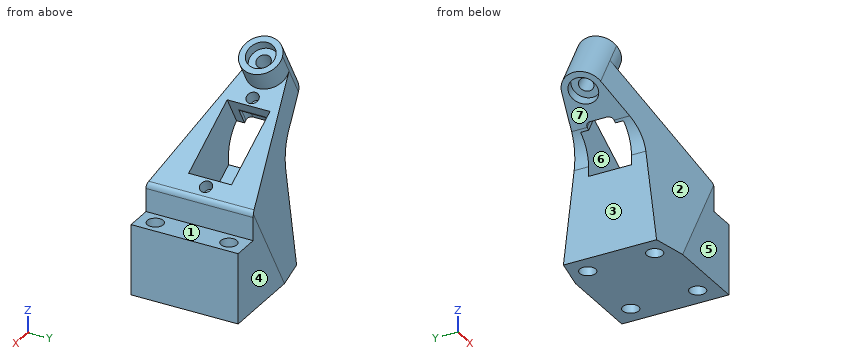
Autodesk Fusion 360 part; units mm, degrees
sketch "Main" plane through (0, 0, 0) normal (0, 1, 0) x (1, 0, 0)
  line L0 (0, 0) -> (35, 0)
  line L1 (35, 0) -> (35, -21)
  line L2 (-19.4678, -44.3397) -> (-14.4678, -53)
  line L3 (-19.4678, -44.3397) -> (0, -33.1)
  line L4 (0, -33.1) -> (0, 0)
  line L5 (-14.4678, -53) -> (27, -29.0585)
  line L6 (35, -21) -> (27, -21)
  line L7 (27, -21) -> (27, -29.0585)
  dimension "d1" = 35
  dimension "d2" = 21
  dimension "d4" = 10
  dimension "d5" = 60
  dimension "d7" = 53
  dimension "d34" = 33.1
  dimension "d35" = 8
extrude "Extrude1" add sketch "Main" along normal blind 32
sketch "Upper Cut " plane through (19.3327, 0, 33.4853) normal (0.5, 0, 0.866) x (0, 1, 0)
  line L0 (0, 39.0295) -> (0, -8.8534)
  line L1 (32, -8.8534) -> (32, 39.0295)
  line L2 (32, 39.0295) -> (0, 39.0295)
  line L3 (0, -30.3109) -> (32, -30.3109) construction
  line L4 (16, 39.0295) -> (16, -30.3109) construction
  arc A0 (21.8411, 34.4013) -> (10.1589, 34.4013) centre (16, 33.0295) ccw
  line L5 (10.1589, 34.4013) -> (0, -8.8534)
  line L6 (21.8411, 34.4013) -> (32, -8.8534)
  line L7 (0, -8.8534) -> (32, -8.8534)
  dimension "d11" = 6
extrude "Extrude2" cut sketch "Upper Cut " against normal blind 43 contours L0 L2 A0 L5 | L1 L2 A0 L6
sketch "Tube Extension" plane through (19.3327, 0, 33.4853) normal (0.5, 0, 0.866) x (0, 1, 0)
  line L0 (32, -8.8534) -> (21.8411, 34.4013)
  arc A0 (21.8411, 34.4013) -> (10.1589, 34.4013) centre (16, 33.0295) ccw
  line L1 (10.1589, 34.4013) -> (0, -8.8534)
  circle A1 centre (16, 33.0295) radius 6
  line L2 (0, -8.8534) -> (32, -8.8534)
  dimension "d14" = 12
extrude "Extrude3" add sketch "Tube Extension" along normal blind 7 contours A0 A1
sketch "Tube Hole" plane through (22.8327, 0, 39.5474) normal (0.5, 0, 0.866) x (0, 1, 0)
  circle A0 centre (16, 33.0295) radius 6
  circle A1 centre (16, 33.0295) radius 2.1
  dimension "d17" = 4.2
extrude "Extrude4" cut sketch "Tube Hole" against normal up to surface (17 mm away) contours A1
fillet "Fillet1" radius 10 1 edges at (0, 16, 33.1)
sketch "Servo Holes" plane through (19.3327, 0, 33.4853) normal (0.5, 0, 0.866) x (0, 1, 0)
  arc A0 (10.1589, 34.4013) -> (21.8411, 34.4013) centre (16, 33.0295) ccw
  line L0 (10.1589, 34.4013) -> (0, -8.8534)
  line L1 (32, -8.8534) -> (21.8411, 34.4013)
  line L2 (16, 27.0295) -> (16, -8.8534) construction
  line L3 (9.6, 21.4466) -> (22.4, 21.4466)
  line L4 (22.4, 21.4466) -> (22.4, -2.3534)
  line L5 (22.4, -2.3534) -> (9.6, -2.3534)
  line L6 (9.6, -2.3534) -> (9.6, 21.4466)
  circle A1 centre (16, 23.9466) radius 1.8
  circle A2 centre (16, -4.8534) radius 1.8
  line L7 (0, -8.8534) -> (32, -8.8534)
  dimension "d22" = 12.8
  dimension "d23" = 23.8
  dimension "d24" = 6.4
  dimension "d28" = 3.6
  dimension "d29" = 3.6
  dimension "d30" = 28.8
  dimension "d31" = 2.5
  dimension "d36" = 6.5
extrude "Extrude5" cut sketch "Servo Holes" against normal blind 17.5 contours L3 L4 L5 L6
extrude "Extrude6" cut sketch "Servo Holes" against normal blind 4 contours A1 | A2
fillet "Fillet3" radius 2 1 edges at (27, 16, 29.0585)
sketch "Top Plate Holes" plane through (0, 0, 21) normal (0, 0, 1) x (-1, 0, 0)
  line L0 (-27, 0) -> (-35, 0)
  line L1 (-35, 0) -> (-35, -32)
  line L2 (-35, -32) -> (-27, -32)
  line L3 (-27, -32) -> (-27, 0)
  line L4 (-31, -32) -> (-31, 0) construction
  circle A0 centre (-31, -27) radius 2.4
  circle A1 centre (-31, -5) radius 2.4
  dimension "d41" = 4.8
  dimension "d42" = 4.8
  dimension "d44" = 22
  dimension "d45" = 5
extrude "Extrude7" cut sketch "Top Plate Holes" against normal blind 8 contours A0 | A1
sketch "Base Holes" plane through (0, 0, 0) normal (0, 0, -1) x (1, 0, 0)
  line L0 (10.223, 0) -> (0, -2.0793)
  line L1 (0, -2.0793) -> (0, -29.9207)
  line L2 (0, -29.9207) -> (10.223, -32)
  line L3 (10.223, -32) -> (35, -32)
  line L4 (35, -32) -> (35, 0)
  line L5 (35, 0) -> (10.223, 0)
  circle A0 centre (6, -6) radius 2.4
  circle A1 centre (29, -6) radius 2.4
  circle A2 centre (6, -26) radius 2.4
  circle A3 centre (29, -26) radius 2.4
  dimension "d59" = 4.8
  dimension "d61" = 6
  dimension "d62" = 6
  dimension "d65" = 23
  dimension "d66" = -20
extrude "Extrude8" cut sketch "Base Holes" against normal blind 8 contours A0 | A1 | A2 | A3
sketch "Servo Wires " plane through (-18.5733, 0, 10.7233) normal (0.866, 0, -0.5) x (0, 1, 0)
  line L0 (9.6, 28.6269) -> (22.4, 28.6269)
  line L1 (22.4, 28.6269) -> (22.4, 38.6654)
  line L2 (22.4, 38.6654) -> (9.6, 38.6654)
  line L3 (9.6, 38.6654) -> (9.6, 28.6269)
  line L4 (12, 33.6269) -> (20, 33.6269)
  line L5 (20, 33.6269) -> (20, 28.6269)
  line L6 (20, 28.6269) -> (12, 28.6269)
  line L7 (12, 28.6269) -> (12, 33.6269)
  dimension "d93" = 8
  dimension "d94" = 2.4
  dimension "d95" = 5
extrude "Extrude9" cut sketch "Servo Wires " against normal blind 2.3 contours L0 L4 L5 L6 L7
fillet "Fillet4" radius 1.4 3 edges at (-1.7598, 16, 39.8451) (-4.9921, 12, 38.8467) (-4.9921, 20, 38.8467)
sketch "Sketch11" plane through (22.8327, 0, 39.5474) normal (0.5, 0, 0.866) x (0, 1, 0)
  circle A0 centre (16, 33.0295) radius 2.1
  circle A1 centre (16, 33.0295) radius 6
  circle A2 centre (16, 33.0295) radius 4.15
  dimension "d100" = 8.3
extrude "Extrude10" cut sketch "Sketch11" against normal blind 3 contours A2
sketch "Sketch12" plane through (14.3327, 0, 24.825) normal (-0.5, 0, -0.866) x (0, -1, 0)
  line L0 (-12, 22.3466) -> (-12, 22.3235)
  line L1 (-12, 22.3235) -> (-7.3223, 22.3235)
  line L2 (-7.3223, 22.3235) -> (-10.1589, 34.4013)
  arc A0 (-10.1589, 34.4013) -> (-21.8411, 34.4013) centre (-16, 33.0295) ccw
  line L3 (-21.8411, 34.4013) -> (-24.6777, 22.3235)
  line L4 (-24.6777, 22.3235) -> (-20, 22.3235)
  line L5 (-20, 22.3235) -> (-20, 22.3466)
  arc A1 (-18.6, 23.7466) -> (-20, 22.3466) centre (-18.6, 22.3466) ccw
  line L6 (-18.6, 23.7466) -> (-13.4, 23.7466)
  arc A2 (-12, 22.3466) -> (-13.4, 23.7466) centre (-13.4, 22.3466) ccw
  circle A3 centre (-16, 33.0295) radius 2.1
  circle A4 centre (-16, 33.0295) radius 4.15
  dimension "d103" = 8.3
extrude "Extrude11" cut sketch "Sketch12" against normal blind 3 contours A4
Input: part model. Units: mm. Frame: model coordinates. Face numbers are marked on the shaded views. A direction names the side the tool comes from. Coordinates: 2 decimals unless noted, no trailing zeros. Order: outer loops, then holes, each group sorted by start corner. A loop starts at its lowest first (then second) coordinate and runs counter-clockwise, first axis right, second up. Notation, with made-up numbers: M 27.5,38 L 45.5,38 A28 cw 45.5,57 Z; hole C 58,4 d5. An arc over 180 degrees is marked long. Answer as CSV lines item,"result".
1. Section A-A (x = 2). Return the cut outline in (y, z).
Reported:
outline,"M 1.67,0 L 30.33,0 L 25.22,43.49 L 22.4,43.49 L 22.4,23.29 L 9.6,23.29 L 9.6,43.49 L 6.78,43.49 Z"
2. Pull-direction query (Y, two-part tool) for the marked faces 4, 5, 6 and 7; classes: released by +Y, released by -Y, zero draft, split by the parting line, or undercut.
Reported:
face 4,"released by +Y"
face 5,"released by -Y"
face 6,"undercut"
face 7,"zero draft"
3. Access query for the marked faces 1, 2 and 3. Directions: +Z, -Z, +X, -X, +Y, -Y. A direction counts if a zero-diameter tool reaches every point of the face in a straight line with its end or side. Return the directions, or none.
Reported:
face 1,"+Z, +X, +Y, -Y"
face 2,"+Z, -X, -Y"
face 3,"-Z, -X, +Y, -Y"
4. First-contact query: P1, Ø4.5, axis at x = 6, y = 6, coming from the -Z side; P2, Ø1.2, axis at x = -2.5, z = 37.5, coming from the +Y side; P3, Ø13, axis at x = 13.5, z = 28.5, coming from the +Y side. Flat tips, straight axial feed; report the tip coordinate or a pass-through.
Reported:
P1,"z = 8"
P2,"y = 25.15"
P3,"y = 30.85"
5. Section B-B (y = 6). Return the cut outline in (x, z).
Reported:
outline,"M -0.99,31.67 A10 cw 0,27.33 L 0,0 L 3.6,0 L 3.6,8 L 8.4,8 L 8.4,0 L 26.6,0 L 26.6,8 L 31.4,8 L 31.4,0 L 35,0 L 35,21 L 33.18,21 L 33.18,13 L 28.82,13 L 28.82,21 L 27,21 L 27,27.9 A2 ccw 26,29.64 L 4.88,41.83 Z"
6. Material intervals for line 1 (Y direction, x = 31, z = 18.75); line 2 (Y direction, x = 29, z = 1); line 3 (X direction, y = 6, z = 4), sorted ascending. Write a range as from..to.
Reported:
line 1,"0..2.6, 7.4..24.6, 29.4..32"
line 2,"0..3.6, 8.4..23.6, 28.4..32"
line 3,"0..3.6, 8.4..26.6, 31.4..35"
